Can you work these out from the model? Positions are in its coordinate system, mm. Round coordinates to 2 decimals unless told otherwise and drop trailing zeros. Order: outer loops, then holes, each group sorted by start corner. A loop starts at its lowest first (then second) coordinate and runs counter-clockwise, first axis right, second up.
Q1. If we section it at A-A (z = 11.5): Please give me the cut outline in (x, y), plus the area to 3 significant figures.
Q2. If we section it at C-C (x = 3.5): Please give me the cut outline in (y, z), plus the area to 3 significant figures.
Q3. If we section it at B-B (y = 5.5): Please give me the cut outline in (x, z), plus the area to 3 significant figures.
Q4. If I drill on line 1 (Y direction, x = 0, z = 19); line 2 (X direction, y = 16.5, z = 4.75); line 3 (X direction, y = 7, z = 20.75), over which ranges is the centre line in solid material (lowest first)?
from build123d import *

# Parameters (mm, degrees)
F0_W     = 50
F0_H     = 60
F0_R     = 19.5
F1_DEPTH = 25
F2_R     = 15
F3_R     = 15


with BuildPart() as f1:
    # F0 (on Top) → F1 (new body)
    with BuildSketch(Plane.XY):
        Rectangle(F0_W, F0_H)
        with Locations((0, 5.5)):
            Circle(F0_R, mode=Mode.SUBTRACT)
    extrude(amount=F1_DEPTH)

    # F2
    f2_edges = [f1.edges().sort_by_distance(p)[0] for p in [
        (-25, 30, 12.5),
    ]]
    fillet(f2_edges, radius=F2_R)

    # F3
    f3_edges = [f1.edges().sort_by_distance(p)[0] for p in [
        (25, 30, 12.5),
    ]]
    fillet(f3_edges, radius=F3_R)


solid = f1.part
Solution:
1. outline: (-25, -30) - (25, -30) - (25, 15) arc R15 ccw to (10, 30) - (-10, 30) arc R15 ccw to (-25, 15) - close; hole circle Ø39 at (0, 5.5)
1. area: 1,710 mm2
2. outline: (-30, 0) - (-13.68, 0) - (-13.68, 25) - (-30, 25) - close; (24.68, 0) - (30, 0) - (30, 25) - (24.68, 25) - close
2. area: 541 mm2
3. outline: (-25, 0) - (-19.5, 0) - (-19.5, 25) - (-25, 25) - close; (19.5, 0) - (25, 0) - (25, 25) - (19.5, 25) - close
3. area: 275 mm2
4. line 1: y = -30 to -14, 25 to 30
4. line 2: x = -24.92 to -16.1, 16.1 to 24.92
4. line 3: x = -25 to -19.44, 19.44 to 25
